from build123d import *

# Parameters (mm, degrees)
F1_DEPTH = 25
F2_SIZE  = 4.99999


# Not quite as in the source:
# - a fillet or chamfer is up to 0.001 mm smaller than in the source, because OpenCascade refuses the exact size


with BuildPart() as f1:
    # F0 (on Front) → F1 (new body)
    with BuildSketch(Plane.XZ):
        Polygon((0, 22.7573593129), (0, 0), (-22.7573593129, 0), (-27, 0), (-32, 0), (-32, -5), (-57, -5), (-57, 0), (-60, 0), (-60, -8), (-29, -8), (-29, -3), (0, -3), (3, -3), (3, 57), (60, 57), (60, 60), (0, 60), (0, 27), align=None)
        Polygon((-22.7573593129, 0), (0, 22.7573593129), (0, 27), (-27, 0), align=None)
    extrude(amount=F1_DEPTH)

    # F2 (size 5 in the source; OpenCascade refuses exactly that, so slightly less here)
    f2_edges = [f1.edges().sort_by_distance(p)[0] for p in [
        (-57, -12.5, -5),
        (-60, -12.5, -8),
        (-29, -12.5, -3),
        (-32, -12.5, 0),
    ]]
    chamfer(f2_edges, length=F2_SIZE)


solid = f1.part
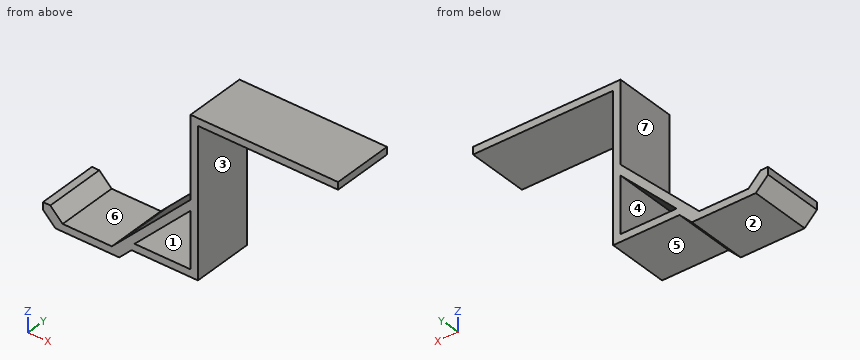
CAD build for the part. Positions are in the model's coordinates, mm. Face numbers are marked on the shaded views. A direction names the side the tool comes from. Coordinates: 2 decimals unless noted, no trailing zeros. Write each loop counter-clockwise with the first axis right and the second up, starting at its lowest first coordinate (ties: lowest second). Pieces come first, ordered by that corner, then holes. Notation, with made-up numbers: (84.25, 13) - (91.25, 13) arc R19 cw to (91.25, 46) - close; hole circle Ø9 at (-24, -11.75). An arc over 180 degrees is marked (long way). Use a Markdown table: item, result. Add a question column.
Item 1: Mould opens along X. For the marked faces 1, 2 and 3 say: pulls with the +X half, pulls with the -X half, needs draft (parallel to the pull), parting line crosses it, or undercut.
Item 2: 3-axis set-ups, long thin cutter, end or side, ignore diameter. For the marked faces 4, 5, 6 and 7: which of +Z, -Z, +X, -X, +Y, -Y reach the whole face in a straight line?
Item 3: Band-saw the part on C-C, the plane x = -15.5. Give the cut face in (y, z).
Item 4: Band-saw the part on B-B, the plane z = 9.5. Give the cut face in (x, y), and give its area (3 significant figures).
Item 5: Band-saw the part on D-D, the plane x = 26. Give the cut face in (y, z).
Item 6: Drill centre lines: L1, parallel to X at y = -2.25, z = 44; L2, parallel to X at y = -4, z = 2; L3, parallel to X at y = -14.25, z = 22. Where is each one in solid material? Low to high. Write a range as from..to.
Item 7: Flat gauge pins, fed straight in: pin 1 (8 mm diameter, centred on y = -17.5, z = 14, fed in from +X); pin 2 (12.5 mm diameter, centred on x = -9.5, y = -10.5, fed in from -Z); pin 3 (2 mm diameter, centred on y = -4, z = 9, fed in from -X). Where does each tip first touch, or does it go through?
Numbers:
| question | item | result |
|---|---|---|
| 1 | face 1 | undercut |
| 1 | face 2 | needs draft |
| 1 | face 3 | pulls with the +X half |
| 2 | face 4 | +Y, -Y |
| 2 | face 5 | -Z, +X, +Y, -Y |
| 2 | face 6 | +Z, +Y, -Y |
| 2 | face 7 | +Z, -X, +Y, -Y |
| 3 | outline | (-25, -3) - (0, -3) - (0, 0) - (-25, 0) - close; (-25, 7.26) - (0, 7.26) - (0, 11.5) - (-25, 11.5) - close |
| 4 | outline | (-17.5, -25) - (-13.26, -25) - (-13.26, 0) - (-17.5, 0) - close; (0, -25) - (3, -25) - (3, 0) - (0, 0) - close |
| 4 | area | 181 mm2 |
| 5 | outline | (-25, 57) - (0, 57) - (0, 60) - (-25, 60) - close |
| 6 | L1 | 0..3 |
| 6 | L2 | -25..-20.76, 0..3 |
| 6 | L3 | -5..-0.76, 0..3 |
| 7 | pin 1 | x = 3 |
| 7 | pin 2 | z = -3 |
| 7 | pin 3 | x = -19 |
